Source: CAD feature listing. Evaluate the final solid. Frame: model axes, mm. A direction names the side the tool comes from. Give positions to 0.01 mm unless a question says otherwise; leave off trailing zeros. Loops run counter-clockwise (first coordinate to the right, second up) from the corner with the lowest first, then second, coordinate; pieces in that order, holes last. Notation, with made-up numbers: (5, 79.5) -> (9, 79.5) arc R19 cw to (9, 104.5) -> close; hole circle Ø7 at (-8, 9.5). An arc over 180 degrees is marked (long way). Put each result on its own line as item: value.
```python
from build123d import *

# Parameters (mm, degrees)
SKETCH1_R            = 8.3
BOSS_EXTRUDE1_DEPTH  = 20
BOSS_EXTRUDE2_DEPTH  = 8
SKETCH3_R            = 4.6
CUT_EXTRUDE1_DEPTH   = 16
SKETCH4_R            = 5.7
CUT_EXTRUDE2_DEPTH   = 7.3
SKETCH5_R            = 3.1
CUT_EXTRUDE3_DEPTH   = 2
SKETCH7_R            = 6.3
BOSS_EXTRUDE3_DEPTH  = 2.9
SKETCH6_R            = 2
CUT_EXTRUDE4_DEPTH   = 10.5
FILLET1_R            = 2.368
SKETCH9_R            = 14.8
BOSS_EXTRUDE5_DEPTH  = 26.6
SKETCH10_R           = 11.1
CUT_EXTRUDE5_DEPTH   = 7.9
SKETCH11_R           = 13.6
CUT_EXTRUDE6_DEPTH   = 1.2
SKETCH12_R           = 8.4
SKETCH12_R_2         = 6.3
BOSS_EXTRUDE6_DEPTH  = 2.4
CUT_SWEEP2_START     = -31.593597178
CUT_SWEEP2_OUTLINE_R = 1
CUT_SWEEP2_DEPTH     = 24.495000761


with BuildPart() as part:
    # Sketch1 → Boss-Extrude1 (new body)
    with BuildSketch(Plane(origin=(0, 0, 0), x_dir=(1, 0, 0), z_dir=(0, 1, 0))):
        with Locations(Location((0, 0, 0), (0, 0, 270))):
            Circle(SKETCH1_R)
    extrude(amount=BOSS_EXTRUDE1_DEPTH)

    # Sketch2 → Boss-Extrude2 (add)
    with BuildSketch(Plane.XZ):
        Polygon((0, 11.027390142), (-9.55, 5.513695071), (-9.55, -5.513695071), (0, -11.027390142), (9.55, -5.513695071), (9.55, 5.513695071), align=None)
    extrude(amount=BOSS_EXTRUDE2_DEPTH)

    # Sketch3 → Cut-Extrude1 (cut)
    with BuildSketch(Plane(origin=(0, 20, 0), x_dir=(1, 0, 0), z_dir=(0, 1, 0))):
        with Locations(Location((0, 0, 0), (0, 0, 270))):
            Circle(SKETCH3_R)
    extrude(amount=-CUT_EXTRUDE1_DEPTH, mode=Mode.SUBTRACT)

    # Sketch4 → Cut-Extrude2 (cut)
    with BuildSketch(Plane(origin=(0, 20, 0), x_dir=(1, 0, 0), z_dir=(0, 1, 0))):
        with Locations(Location((0, 0, 0), (0, 0, 270))):
            Circle(SKETCH4_R)
    extrude(amount=-CUT_EXTRUDE2_DEPTH, mode=Mode.SUBTRACT)

    # Sketch5 → Cut-Extrude3 (cut)
    with BuildSketch(Plane(origin=(0, 4, 0), x_dir=(1, 0, 0), z_dir=(0, 1, 0))):
        with Locations(Location((0, 0, 0), (0, 0, 270))):
            Circle(SKETCH5_R)
    extrude(amount=-CUT_EXTRUDE3_DEPTH, mode=Mode.SUBTRACT)

    # Sketch7 → Boss-Extrude3 (add)
    with BuildSketch(Plane.XZ.offset(8)):
        with Locations(Location((0, 0, 0), (0, 0, 270))):
            Circle(SKETCH7_R)
    extrude(amount=BOSS_EXTRUDE3_DEPTH)

    # Sketch6 → Cut-Extrude4 (cut)
    with BuildSketch(Plane(origin=(0, 2, 0), x_dir=(1, 0, 0), z_dir=(0, 1, 0))):
        with Locations(Location((0, 0, 0), (0, 0, 270))):
            Circle(SKETCH6_R)
    extrude(amount=-CUT_EXTRUDE4_DEPTH, mode=Mode.SUBTRACT)

    # Fillet1
    # the kernel refuses this fillet: 2.368 mm, written as the material it adds along each edge
    with BuildSketch(Plane(origin=(0, 2, 0), x_dir=(0, 0, 1), z_dir=(-1, 0, 0))) as fillet1_piece_1:
        with BuildLine():
            CenterArc((0.732, 1.999899998), FILLET1_R, 302.375992961, 57.624007039)
            Line((2, 0), (3.1, 0))
            Line((3.1, 0), (3.1, 1.999899998))
        make_face()
    revolve(axis=Axis((0, 2, 0), (0, 1, 0)))

    # Sketch9 → Boss-Extrude5 (add)
    with BuildSketch(Plane.XZ.offset(10.9)):
        with Locations(Location((0, 0, 0), (0, 0, 270))):
            Circle(SKETCH9_R)
    extrude(amount=BOSS_EXTRUDE5_DEPTH)

    # Sketch10 → Cut-Extrude5 (cut)
    with BuildSketch(Plane.XZ.offset(37.5)):
        with Locations(Location((0, 0, 0), (0, 0, 270))):
            Circle(SKETCH10_R)
    extrude(amount=-CUT_EXTRUDE5_DEPTH, mode=Mode.SUBTRACT)

    # Sketch11 → Cut-Extrude6 (cut)
    with BuildSketch(Plane.XZ.offset(37.5)):
        with Locations(Location((0, 0, 0), (0, 0, 270))):
            Circle(SKETCH11_R)
    extrude(amount=-CUT_EXTRUDE6_DEPTH, mode=Mode.SUBTRACT)

    # Sketch12 → Boss-Extrude6 (add)
    with BuildSketch(Plane.XZ.offset(29.6)):
        with Locations(Location((0, 0, 0), (0, 0, 270))):
            Circle(SKETCH12_R)
        with Locations(Location((0, 0, 0), (0, 0, 270))):
            Circle(SKETCH12_R_2, mode=Mode.SUBTRACT)
    extrude(amount=BOSS_EXTRUDE6_DEPTH)

    # Cut-Sweep2: read off the stored shape, not the designer's step
    # Cut-Sweep2 outline → Cut-Sweep2 (cut)
    with BuildSketch(Plane(origin=(0, 0, 0), x_dir=(1, 0, 0), z_dir=(0, 0.9247029674801356, -0.38068940349506886)).offset(CUT_SWEEP2_START)):
        with Locations((0, 2.012129639)):
            Circle(CUT_SWEEP2_OUTLINE_R)
    extrude(amount=CUT_SWEEP2_DEPTH, mode=Mode.SUBTRACT)


solid = part.part
```
(1) First-contact query: P1, Ø7.5, axis at x = 0, z = 0, coming from the +Y side; P2, Ø2.5, axis at y = -2.5, z = 1, coming from the -X side; P3, Ø5, axis at x = 1.5, z = -1.5, coming from the -Y side. Flat tips, straight axial feed; report the tip coordinate or a pass-through.
Calculated:
P1: stops at y = 4
P2: stops at x = -9.55
P3: stops at y = -29.6
(2) Section A-A on y = -1. Return loops of the section in (x, z).
Calculated:
outline: (-9.55, -5.51) -> (0, -11.03) -> (9.55, -5.51) -> (9.55, 5.51) -> (0, 11.03) -> (-9.55, 5.51) -> close; hole circle Ø4 at (0, 0)
(3) Section B-B on z = -9.5. Return loops of the section in (x, y), then the cut area to 3 significant figures.
Calculated:
outline: (-11.35, -37.5) -> (-9.73, -37.5) -> (-9.73, -36.3) -> (-5.74, -36.3) -> (-5.74, -29.6) -> (5.74, -29.6) -> (5.74, -36.3) -> (9.73, -36.3) -> (9.73, -37.5) -> (11.35, -37.5) -> (11.35, -10.9) -> (-11.35, -10.9) -> close; (-2.65, -8) -> (2.65, -8) -> (2.65, 0) -> (-2.65, 0) -> close
area: 546 mm²
(4) Reachability of faces 1 (the flat face through (-3, 0, -8)), 2 (the flat face through (-4.38, -8, -4.75)), 3 (the cylindrical face through (-13.277, -36.908, 2.948)) from +Z, -Z, +X, -X, +Y, -Y: full face, straight path, thin tool, end or side. Return the list, or none.
Calculated:
face 1: +Y
face 2: none
face 3: -Y
(5) Draft query along Z for faces 4 (the cylindrical face through (-14.448, -24.014, 3.208)), 5 (the flat face through (-8.2, -29.6, 2.5)), 6 (the flat face through (6, 20, 2)). Return one class per face: released by +Z, released by -Z, zero draft, split by the parting line, or undercut.
Calculated:
face 4: split by the parting line
face 5: undercut
face 6: zero draft
(6) Section C-C on z = 7.5. Give the number of separate pieces and of enclosed holes in the cut face, then the cut area to 3 significant figures.
Calculated:
separate pieces: 2
enclosed holes: 1
area: 792 mm²
(7) Section D-D on y = 10. Return loops of the section in (x, z).
Calculated:
outline: circle Ø16.6 at (0, 0); hole circle Ø9.2 at (0, 0)
(8) Line query: probe 1 along X at (y, z) = (-31.35, 0); probe 2 along X at (y, z) = (-30.5, 6.75); probe 3 along Y at (x, z) = (-3.75, 8.75). Output: solid intervals per line, ascending. Write a range as from..to.
Calculated:
probe 1: x = -14.8..-11.1, -8.4..-6.3, 6.3..8.4, 11.1..14.8
probe 2: x = -13.17..-8.81, -5..5, 8.81..13.17
probe 3: y = -29.6..-10.9, -8..0
